Could you check a few things on this model? Use its own coordinates, in mm. Face numbers are marked on the shaded views. A direction names the side the tool comes from. Give positions to 0.01 mm unless a question says otherwise; leave off trailing zeros. Loops run counter-clockwise (first coordinate to the right, second up) from the corner with the lowest first, then second, coordinate; pieces in that order, holes last. Notation, with made-up numbers: M 55.25,-24.75 L 74.25,-24.75 A10 ccw 74.25,-19.75 Z; hole C -16,-11 d6. An arc over 180 degrees is marked long. Answer in a Markdown table with one row per item. Add a question column.
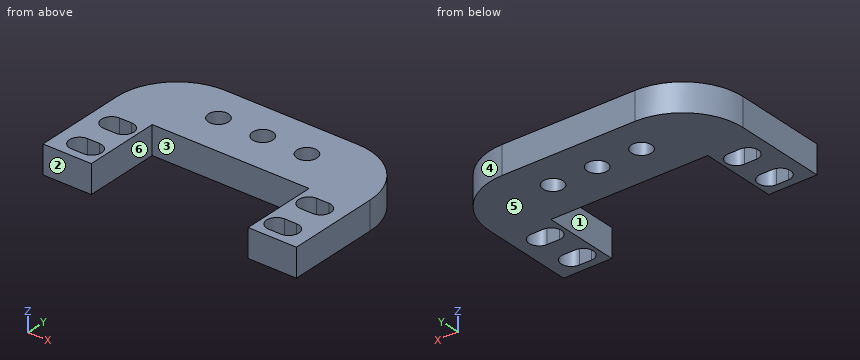
```python
from build123d import *

# Parameters (mm, degrees)
SKETCH_R    = 2.5
PAD_DEPTH   = 7
FILLET_R    = 15
FILLET001_R = 15


with BuildPart() as part:
    # Sketch → Pad (new body)
    with BuildSketch(Plane.XY):
        Polygon((-31.5, 19), (31.5, 19), (31.5, -19), (19.5, -19), (19.5, 0), (-19.5, 0), (-19.5, -19), (-31.5, -19), align=None)
        with Locations((-11, 10)):
            Circle(SKETCH_R, mode=Mode.SUBTRACT)
        with Locations((0, 10)):
            Circle(SKETCH_R, mode=Mode.SUBTRACT)
        with Locations((11, 10)):
            Circle(SKETCH_R, mode=Mode.SUBTRACT)
        with BuildLine():
            ThreePointArc((-26, -2), (-28.5, -4.5), (-26, -7))
            Line((-26, -7), (-23, -7))
            ThreePointArc((-23, -7), (-20.5, -4.5), (-23, -2))
            Line((-23, -2), (-26, -2))
        make_face(mode=Mode.SUBTRACT)
        with BuildLine():
            ThreePointArc((-26, -12), (-28.5, -14.5), (-26, -17))
            Line((-26, -17), (-23, -17))
            ThreePointArc((-23, -17), (-20.5, -14.5), (-23, -12))
            Line((-23, -12), (-26, -12))
        make_face(mode=Mode.SUBTRACT)
        with BuildLine():
            ThreePointArc((23, -2), (20.5, -4.5), (23, -7))
            Line((23, -7), (26, -7))
            ThreePointArc((26, -7), (28.5, -4.5), (26, -2))
            Line((26, -2), (23, -2))
        make_face(mode=Mode.SUBTRACT)
        with BuildLine():
            ThreePointArc((23, -12), (20.5, -14.5), (23, -17))
            Line((23, -17), (26, -17))
            ThreePointArc((26, -17), (28.5, -14.5), (26, -12))
            Line((26, -12), (23, -12))
        make_face(mode=Mode.SUBTRACT)
    extrude(amount=PAD_DEPTH)

    # Fillet
    fillet_edges = [part.edges().sort_by_distance(p)[0] for p in [
        (-31.5, 19, 3.5),
    ]]
    fillet(fillet_edges, radius=FILLET_R)

    # Fillet001
    fillet001_edges = [part.edges().sort_by_distance(p)[0] for p in [
        (31.5, 19, 3.5),
    ]]
    fillet(fillet001_edges, radius=FILLET001_R)


solid = part.part
```
Item 1: For the marked faces 5 and 6, which set-ups out of +Z, -Z, +X, -X, +Y, -Y let a thin tool reach every point of the face, with its end or its side?
Item 2: Suppose I cut it at B-B (x = 0). List the corners of the cut face in (y, z) for me, then the cut area to 3 significant figures.
Item 3: For P1, Ø2.5, axis at x = -24, z = 3.5, coming from the +Y side; P2, Ø1.5, axis at y = 10.5, z = 4, coming from the -X side; P3, Ø0.9, axis at x = 25, z = 4.5, coming from the +Y side; P4, Ø10, axis at x = 8, y = 0.5, coming from the -Z side, each with a flat end and sliding along its axis, tell me the tip position at first contact or that it passes through.
Item 4: If we mould it in two halves opening along X, with no side actions, what happens to the marked faces 1, 2, 3 and 4? For each: +X half, -X half, draft (parallel to the pull), parting line (faces both ways), or undercut.
Item 5: Suppose I cut it at D-D (y = 10). List the corners of the cut face in (x, z) for me.
Item 6: Suppose I cut it at C-C (z = 1). Give the number of separate pieces and of enclosed holes in the cut face, then the cut area to 3 significant figures.
Item 7: I need wall thicknesses on L1, parallel to Y at x = 0, z = 4; L2, parallel to X at y = -13.5, z = 0.5; L3, parallel to Y at x = 24, z = 6.25. Which ranges of each line are inside material? Lowest first, please.
Item 8: Suppose I cut it at A-A (y = -14.5). List the corners of the cut face in (x, z) for me, then the cut area to 3 significant figures.
Values found:
| question | item | result |
|---|---|---|
| 1 | face 5 | -Z, +X, -X, +Y, -Y |
| 1 | face 6 | +Z, -Z, -Y |
| 2 | outline | M 0,0 L 7.5,0 L 7.5,7 L 0,7 Z; M 12.5,0 L 19,0 L 19,7 L 12.5,7 Z |
| 2 | area | 98.0 mm² |
| 3 | P1 | y = 17.64 |
| 3 | P2 | x = -30.35 |
| 3 | P3 | y = 16.66 |
| 3 | P4 | z = 0 |
| 4 | face 1 | undercut |
| 4 | face 2 | draft |
| 4 | face 3 | undercut |
| 4 | face 4 | +X half |
| 5 | outline | M -30.25,0 L -13.5,0 L -13.5,7 L -30.25,7 Z; M -8.5,0 L -2.5,0 L -2.5,7 L -8.5,7 Z; M 2.5,0 L 8.5,0 L 8.5,7 L 2.5,7 Z; M 13.5,0 L 30.25,0 L 30.25,7 L 13.5,7 Z |
| 6 | separate pieces | 1 |
| 6 | enclosed holes | 7 |
| 6 | area | 1,360 mm² |
| 7 | L1 | 0 to 7.5, 12.5 to 19 |
| 7 | L2 | -31.5 to -28.29, -20.71 to -19.5, 19.5 to 20.71, 28.29 to 31.5 |
| 7 | L3 | -19 to -17, -12 to -7, -2 to 16.99 |
| 8 | outline | M -31.5,0 L -28.5,0 L -28.5,7 L -31.5,7 Z; M -20.5,0 L -19.5,0 L -19.5,7 L -20.5,7 Z; M 19.5,0 L 20.5,0 L 20.5,7 L 19.5,7 Z; M 28.5,0 L 31.5,0 L 31.5,7 L 28.5,7 Z |
| 8 | area | 56.0 mm² |
